```python
from build123d import *

# Parameters (mm, degrees)
SKETCH1_W           = 25
SKETCH1_H           = 50
SKETCH1_R           = 3.1
BOSS_EXTRUDE1_DEPTH = 3
SKETCH2_W           = 50
SKETCH2_H           = 3
BOSS_EXTRUDE2_DEPTH = 8
SKETCH3_W           = 8
SKETCH3_H           = 50
BOSS_EXTRUDE3_DEPTH = 42
SKETCH4_R           = 2.65
CUT_EXTRUDE1_DEPTH  = 3.3
FILLET1_R           = 1
SKETCH5_R           = 3.868246804
CUT_EXTRUDE2_DEPTH  = 9
FILLET2_R           = 1
SKETCH6_R           = 12.5
BOSS_EXTRUDE4_DEPTH = 2
FILLET3_R           = 1
FILLET4_R           = 1


with BuildPart() as part:
    # Sketch1 → Boss-Extrude1 (new body)
    with BuildSketch(Plane(origin=(0, 0, 0), x_dir=(1, 0, 0), z_dir=(0, 1, 0))):
        with Locations((2.276951673, 11.384758364)):
            Rectangle(SKETCH1_W, SKETCH1_H)
        with Locations(Location((1.276951673, 11.384758364, 0), (0, 0, 270))):
            Circle(SKETCH1_R, mode=Mode.SUBTRACT)
    extrude(amount=BOSS_EXTRUDE1_DEPTH)

    # Sketch2 → Boss-Extrude2 (add)
    with BuildSketch(Plane.ZY.offset(10.223048327)):
        with Locations((-11.384758364, 1.5)):
            Rectangle(SKETCH2_W, SKETCH2_H)
    extrude(amount=BOSS_EXTRUDE2_DEPTH)

    # Sketch3 → Boss-Extrude3 (add)
    with BuildSketch(Plane.XZ):
        with Locations((-14.223048327, -11.384758364)):
            Rectangle(SKETCH3_W, SKETCH3_H)
    extrude(amount=BOSS_EXTRUDE3_DEPTH)

    # Sketch4 → Cut-Extrude1 (cut)
    with BuildSketch(Plane(origin=(0, 3, 0), x_dir=(1, 0, 0), z_dir=(0, 1, 0))):
        with Locations(Location((-14.223048327, 32.384758364, 0), (0, 0, 270))):
            Circle(SKETCH4_R)
        with Locations(Location((-14.223048327, -9.615241636, 0), (0, 0, 270))):
            Circle(SKETCH4_R)
    cut_extrude1 = extrude(amount=-CUT_EXTRUDE1_DEPTH, mode=Mode.SUBTRACT)

    # Mirror1: Cut-Extrude1 across plane
    add(cut_extrude1.mirror(Plane.ZX.offset(-19.5)), mode=Mode.SUBTRACT)

    # Fillet1
    fillet1_edges = [part.edges().sort_by_distance(p)[0] for p in [
        (1.276951673, 0, -14.484758364),
    ]]
    fillet(fillet1_edges, radius=FILLET1_R)

    # Sketch5 → Cut-Extrude2 (cut)
    with BuildSketch(Plane.ZY.offset(18.223048327)):
        with Locations((-11.836279124, -21)):
            Circle(SKETCH5_R)
    extrude(amount=-CUT_EXTRUDE2_DEPTH, mode=Mode.SUBTRACT)

    # Fillet2
    fillet2_edges = [part.edges().sort_by_distance(p)[0] for p in [
        (-10.223048327, -21, -15.704525928),
    ]]
    fillet(fillet2_edges, radius=FILLET2_R)

    # Mirror2: Cut-Extrude1 across plane
    add(cut_extrude1.mirror(Plane.ZY.offset(1.723048327)), mode=Mode.SUBTRACT)

    # Sketch6 → Boss-Extrude4 (add)
    with BuildSketch(Plane(origin=(0, 3, 0), x_dir=(1, 0, 0), z_dir=(0, 1, 0))):
        with BuildLine():
            Line((14.776951673, 6.093255742), (14.776951673, 16.676260986))
            ThreePointArc((14.776951673, 16.676260986), (-13.223048327, 11.384758364), (14.776951673, 6.093255742))
        make_face()
        with Locations(Location((1.276951673, 11.384758364, 0), (0, 0, 270))):
            Circle(SKETCH6_R, mode=Mode.SUBTRACT)
    extrude(amount=BOSS_EXTRUDE4_DEPTH)

    # Fillet3
    fillet3_edges = [part.edges().sort_by_distance(p)[0] for p in [
        (-10.223048327, 0, -11.384758364),
    ]]
    fillet(fillet3_edges, radius=FILLET3_R)

    # Fillet4
    fillet4_edges = [part.edges().sort_by_distance(p)[0] for p in [
        (14.776951673, 5, -11.384758364),
    ]]
    fillet(fillet4_edges, radius=FILLET4_R - 0.0001)  # a hair under: the kernel refuses the full size


solid = part.part
```
The listing builds one solid part. Answer for the finished solid, in the listing's coordinates (mm). A direction names the side the tool comes from. Round coordinates to 2 decimals unless told otherwise and drop trailing zeros. Write each loop counter-clockwise with the first axis right and the second up, starting at its lowest first coordinate (ties: lowest second). Pieces come first, ordered by that corner, then holes. Notation, with made-up numbers: (21, -7) -> (63, -7) arc R20 cw to (63, 25) -> close; hole circle Ø6 at (-36.75, 38.25). An arc over 180 degrees is marked (long way). Answer as a JSON object with one key per item and string values. Group by question number.
Q1. Section D-D (y = -11.5) is taken. Write down the section's boundary in (x, z).
Q2. Determine the mould class of faces 5 (the face through (-11.99, 1.37, -30.96)), 6 (the face through (-14, -0.3, 10)), 7 (the face through (14.777, 2, -11)), 8 (the face through (-12, -14, 13.615)) for opening direction Z: pulls with the +Z half, pulls with the -Z half, needs draft (parallel to the pull), parting line crosses it, or undercut.
Q3. Section B-B (x = 9) is taken. Write down the section's boundary in (y, z).
Q4. Straight lines are drawn through the part: line 1 along X through (y, z) = (1.5, -30); line 2 along Y through (x, z) = (12, -8); line 3 along X through (y, z) = (-26, -21). For each, find the intervals that lie inside material, in ascending order.
Q5. Section C-C (z = 2.5) is taken. Write down the section's boundary in (x, y).
Q6. Section A-A (y = -21) is taken. Write down the section's boundary in (x, z), plus the area to 3 significant figures.
Q7. Which of the six approach directions +Z, -Z, +X, -X, +Y, -Y give full straight-line access (tool end or side, diameter ignored) to faces 1 (the face through (-14, -38.7, 10)), 2 (the face through (6, 0, -12)), 3 (the face through (-14, -0.3, -32)), 4 (the face through (-18.223, -14, -12))?
Q8. Each of these flat-tipped pins is pushed along its axis until it touches: pin 1 Ø7 at (x, z) = (10.78, -32.38) entering from +Y; pin 2 Ø4 at (x, z) = (5, -23.5) entering from -Y; pin 3 Ø3 at (x, z) = (-14.22, 9.62) entering from +Y. Where does it stop, or does it pass through?
Check values:
{
 "1": {"outline": "(-18.22, -36.38) -> (-10.22, -36.38) -> (-10.22, 13.62) -> (-18.22, 13.62) -> close"},
 "2": {"face 5": "undercut", "face 6": "undercut", "face 7": "needs draft", "face 8": "pulls with the +Z half"},
 "3": {"outline": "(0, -36.38) -> (3, -36.38) -> (3, -34.35) -> (0, -34.35) -> close; (0, -30.42) -> (3, -30.42) -> (3, -23.66) -> (5, -23.66) -> (5, -21.21) -> (3, -21.21) -> (3, -1.56) -> (5, -1.56) -> (5, 0.89) -> (3, 0.89) -> (3, 7.65) -> (0, 7.65) -> close; (0, 11.58) -> (3, 11.58) -> (3, 13.62) -> (0, 13.62) -> close"},
 "4": {"line 1": "-18.22 to -15.38, -13.07 to 9.62, 11.93 to 14.78", "line 2": "0 to 3", "line 3": "-18.22 to -10.22"},
 "5": {"outline": "(-18.22, -42) -> (-10.22, -42) -> (-10.22, -1) arc R1 cw to (-9.22, 0) -> (14.78, 0) -> (14.78, 3) -> (5.46, 3) -> (5.46, 5) -> (-2.9, 5) -> (-2.9, 3) -> (-18.22, 3) -> close"},
 "6": {"outline": "(-18.22, -36.38) -> (-10.22, -36.38) -> (-10.22, -16.7) arc R1 ccw to (-11.22, -15.7) -> (-18.22, -15.7) -> close; (-18.22, -7.97) -> (-11.22, -7.97) arc R1 ccw to (-10.22, -6.97) -> (-10.22, 13.62) -> (-18.22, 13.62) -> close", "area": "338 mm^2"},
 "7": {"face 1": "-Y", "face 2": "+Z, -Z, +X, -Y", "face 3": "+Y", "face 4": "+Z, -Z, -X, +Y, -Y"},
 "8": {"pin 1": "y = 3", "pin 2": "y = 0", "pin 3": "y = -0.3"}
}
